Check sheet for the modelled part. Datum: model origin and axes. Units: mm. A direction names the side the tool comes from. Round coordinates to 2 decimals unless told otherwise and drop trailing zeros. Write each loop counter-clockwise with the first axis right and the second up, starting at its lowest first coordinate (ties: lowest second). Pieces come first, ordered by that corner, then holes. Notation, with made-up numbers: M 69,-3 L 73,-3 A20 ccw 73,12 Z; hole C 76.25,53 d11. An arc over 180 degrees is marked long. One line per item, written item: value.
from build123d import *

# Parameters (mm, degrees)
PAD_DEPTH       = 10
SKETCH001_R     = 1.25
POCKET_DEPTH    = 22.501
POCKET001_DEPTH = 5
FILLET_R        = 3


with BuildPart() as part:
    # Sketch → Pad (new body)
    with BuildSketch(Plane.XY):
        with BuildLine():
            Line((0, 26), (31.5, 26))
            ThreePointArc((32.5, 25), (32.207107, 25.707107), (31.5, 26))
            Line((32.5, 25), (32.5, 0))
            Line((32.5, 0), (44.5, 0))
            Line((44.5, 22.5), (44.5, 0))
            Line((36.5, 22.5), (44.5, 22.5))
            Line((36.5, 32), (36.5, 22.5))
            ThreePointArc((36.5, 32), (35.035534, 35.535534), (31.5, 37))
            Line((0, 37), (31.5, 37))
            Line((0, 37), (0, 26))
        make_face()
    extrude(amount=PAD_DEPTH)

    # Sketch001 (on Face7 of Pad) → Pocket (cut, through all)
    with BuildSketch(Plane(origin=(0, 22.5, 0), x_dir=(-1, 0, 0), z_dir=(0, 1, 0))):
        with Locations((-40.75, 5)):
            Circle(SKETCH001_R)
    extrude(amount=-POCKET_DEPTH, mode=Mode.SUBTRACT)

    # Sketch002 (on Face5 of Pocket) → Pocket001 (cut)
    with BuildSketch(Plane.XY.offset(10)):
        with BuildLine():
            Line((0, 0), (32.5, 0))
            Line((32.5, 0), (32.5, 32))
            ThreePointArc((32.5, 32), (32.207107, 32.707107), (31.5, 33))
            Line((0, 33), (31.5, 33))
            Line((0, 0), (0, 33))
        make_face()
    extrude(amount=-POCKET001_DEPTH, mode=Mode.SUBTRACT)

    # Fillet
    fillet_edges = [part.edges().sort_by_distance(p)[0] for p in [
        (44.5, 11.25, 10),
        (44.5, 11.25, 0),
    ]]
    fillet(fillet_edges, radius=FILLET_R)

    # Mirrored: part across YZ


with BuildPart() as part_1:
    add(part.part)
    add(part.part.mirror(Plane.YZ))


solid = part_1.part
Q1. Sectioned sample at B-B on x = -16.5. Enter the section's corners in (y, z).
Completed:
outline: M 26,0 L 37,0 L 37,10 L 33,10 L 33,5 L 26,5 Z
Q2. Scan lines: line 1 (X direction, y = 29.5, z = 8.5); line 2 (Z direction, x = -40.75, y = 16); line 3 (X direction, y = 15, z = 6.5). Record each from-to range of solid material in increasing order. Write a range as [from, to].
Completed:
line 1: [-36.5, -32.5], [32.5, 36.5]
line 2: [0, 3.75], [6.25, 10]
line 3: [-44.5, -32.5], [32.5, 44.5]
Q3. Depth check by flat-ended pin: P1, Ø2.5, axis at x = 42, z = 3.5, coming from the +Y side; P2, Ø1, axis at x = 34.5, z = 3, coming from the -Y side; P3, Ø2.5, axis at x = -15.5, y = 29.5, coming from the +Z side; P4, Ø1.5, axis at x = -1, z = 8, coming from the -Y side. Enter the tip coordinate at first touch or a pass-through.
Completed:
P1: y = 22.5
P2: y = 0
P3: z = 5
P4: y = 33
Q4. Access from +Z, -Z, +X, -X, +Y, -Y to the whole of each face (thin tool, end or side, straight path). Record for faces 4 (the flat face through (36.5, 27, 5)), 5 (the flat face through (-39.6, 22.5, 3.8)), 6 (the flat face through (0, 33, 8)), 7 (the flat face through (0, 26, 2)).
Completed:
face 4: +Z, -Z, +X, +Y
face 5: +Z, -Z, -X, +Y
face 6: +Z, -Y
face 7: +Z, -Z, -Y
Q5. Sectioned sample at A-A on y = 10.5. Enter the section's corners in (x, z), and give its area (3 significant figures).
Completed:
outline: M -44.5,3 A3 ccw -41.5,0 L -32.5,0 L -32.5,10 L -41.5,10 A3 ccw -44.5,7 Z; M 32.5,0 L 41.5,0 A3 ccw 44.5,3 L 44.5,7 A3 ccw 41.5,10 L 32.5,10 Z; hole C -40.75,5 d2.5; hole C 40.75,5 d2.5
area: 222 mm^2
Q6. Draft check along Z on faces 1 (the cylindrical face through (-41.74, 11.41, 4.24)), 2 (the flat face through (44.5, 11, 5)), 3 (the cylindrical face through (-43.64, 11.09, 9.1)). Enter one of: pulls with the +Z half, pulls with the -Z half, needs draft (parallel to the pull), parting line crosses it, or undercut.
Completed:
face 1: undercut
face 2: needs draft
face 3: pulls with the +Z half
